from build123d import *

# Parameters (mm, degrees)
SKETCH_1_W                   = 20
SKETCH_1_H                   = 40
EXTRUDE_1_DEPTH              = 5.5
SKETCH_2_W                   = 2
SKETCH_2_H                   = 2
CUT_EXTRUDE_1_DEPTH          = 46.058295574
SKETCH_3_R                   = 2.25
EXTRUDE_2_DEPTH              = 40
SKETCH_3_2_R                 = 2.25
CUT_EXTRUDE_2_DEPTH          = 46.82575695
CHAMFER_1_SIZE               = 2
SKETCH_4_W                   = 9
SKETCH_4_H                   = 10
CUT_EXTRUDE_3_DEPTH          = 31
HOLE_WIZARD_M5_3_D           = 5.3
HOLE_WIZARD_M5_3_DEPTH       = 6
HOLE_WIZARD_M5_3_CSINK_D     = 10.2
HOLE_WIZARD_M5_3_CSINK_ANGLE = 70
HOLE_WIZARD_M5_3_TIP         = 1.59228064


with BuildPart() as part:
    # 草图1 → 凸台-拉伸1 (new body)
    with BuildSketch(Plane(origin=(0, 0, 0), x_dir=(1, 0, 0), z_dir=(0, 1, 0))):
        with Locations((-10, 0)):
            Rectangle(SKETCH_1_W, SKETCH_1_H)
    extrude(amount=EXTRUDE_1_DEPTH)

    # 草图2 → 切除-拉伸1 (cut, through all)
    with BuildSketch(Plane.XY.offset(20)):
        with Locations((-1, 1)):
            Rectangle(SKETCH_2_W, SKETCH_2_H)
    extrude(amount=-CUT_EXTRUDE_1_DEPTH, mode=Mode.SUBTRACT)

    # 草图3 → 凸台-拉伸2 (add)
    with BuildSketch(Plane.XY.offset(20)):
        with BuildLine():
            Line((-1.968626967, 10), (1.968626967, 10))
            Line((1.968626967, 10), (3.968626967, 8))
            Line((3.968626967, 8), (3.968626967, 5.5))
            ThreePointArc((3.968626967, 5.5), (0, 2), (-3.968626967, 5.5))
            Line((-3.968626967, 5.5), (-3.968626967, 8))
            Line((-3.968626967, 8), (-1.968626967, 10))
        make_face()
        with Locations((0, 6)):
            Circle(SKETCH_3_R, mode=Mode.SUBTRACT)
    extrude(amount=-EXTRUDE_2_DEPTH)

    # 草图3<2> → 切除-拉伸2 (cut, through all)
    with BuildSketch(Plane.XY.offset(20)):
        with Locations((0, 6)):
            Circle(SKETCH_3_2_R)
    extrude(amount=-CUT_EXTRUDE_2_DEPTH, mode=Mode.SUBTRACT)

    # 倒角1
    chamfer_1_edges = [part.edges().sort_by_distance(p)[0] for p in [
        (-20, 5.5, 0),
    ]]
    chamfer(chamfer_1_edges, length=CHAMFER_1_SIZE)

    # 草图4 → 切除-拉伸3 (cut, through all)
    with BuildSketch(Plane(origin=(0, 0, 0), x_dir=(1, 0, 0), z_dir=(0, 1, 0))):
        with Locations((-0.531373033, 5)):
            Rectangle(SKETCH_4_W, SKETCH_4_H)
        with Locations((-0.531373033, -15)):
            Rectangle(SKETCH_4_W, SKETCH_4_H)
    extrude(amount=CUT_EXTRUDE_3_DEPTH, mode=Mode.SUBTRACT)

    # M5 十字切槽平头螺钉锥孔槽口3
    with Locations(Plane(origin=(0, 5.5, 0), x_dir=(1, 0, 0), z_dir=(0, 1, 0))):
        with Locations((-12.5, 12.5), (-12.5, -12.5)):
            CounterSinkHole(HOLE_WIZARD_M5_3_D / 2, HOLE_WIZARD_M5_3_CSINK_D / 2, depth=HOLE_WIZARD_M5_3_DEPTH, counter_sink_angle=HOLE_WIZARD_M5_3_CSINK_ANGLE)
            with Locations((0, 0, -(HOLE_WIZARD_M5_3_DEPTH + HOLE_WIZARD_M5_3_TIP / 2))):  # 118° drill point
                Cone(0, HOLE_WIZARD_M5_3_D / 2, HOLE_WIZARD_M5_3_TIP, mode=Mode.SUBTRACT)


solid = part.part
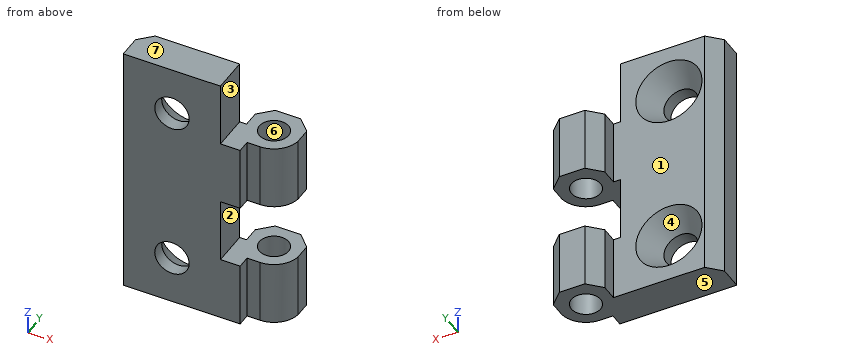
Read the model definition and answer for the solid it produces. Units are mm, in the model's axes. Face numbers are marked on the shaded views. A direction names the side the tool comes from. Give positions to 0.01 mm unless a question says otherwise; leave off trailing zeros. Write each loop counter-clockwise with the first axis right and the second up, starting at its lowest first coordinate (ties: lowest second). Pieces come first, ordered by that corner, then holes. Notation, with made-up numbers: (-12, 33.5) - (42, 33.5) arc R8 ccw to (42, 43.5) - close; hole circle Ø6 at (77.5, 70). An arc over 180 degrees is marked (long way). Use CSV: the item, a comma, the result in double quotes. Start each with the question number.
(1) Consider line 1 along Z through (x, y) = (-12.5, 1.6); line 2 along X through (y, z) = (6, -15.5); line 3 along Y through (x, z) = (0, 3.75). Determine where each line is inside the solid, lowest interval first.
(2) Find section C-C (x = -12.5). Give the vertices of the cut face in (y, z), plus the area to 3 significant figures.
(3) Given P1, Ø11, axis at x = -11.5, z = 5.5, coming from the +Y side; P2, Ø1.6, axis at y = 1.5, z = 6.5, coming from the +X side; P3, Ø1.6, axis at y = 1, z = -17.5, coming from the +X side, each flat-ended and moving along its own axis, determine where each tip first touches the part or whether it passes through.
(4) Find section B-B (y = 6). Give the vertices of the cut face in (x, z).
(5) Determine the mould class of the marked faces 4, 5, 6 and 7 for opening direction Z: +Z half, -Z half, draft (parallel to the pull), parting line (faces both ways), or undercut.
(6) For the marked faces 1, 2 and 3, determine the directions among +Z, -Z, +X, -X, +Y, -Y from which every point of the face is accessible in a straight line to the end or side of a thin tool.
(7) Find section A-A (z = 12.5). Give the vertices of the cut face in (x, y).
(8) Find section D-D (y = 8.75). Give the vertices of the cut face in (x, z), plus the area to 3 significant figures.
Findings below:
1,line 1,"-20 to -15.15, -9.85 to 9.85, 15.15 to 20"
1,line 2,"-3.97 to -2.25, 2.25 to 3.97"
1,line 3,"2 to 3.75, 8.25 to 10"
2,outline,"(0, -20) - (5.5, -20) - (5.5, -17.6) - (2, -15.15) - (0, -15.15) - close; (0, -9.85) - (2, -9.85) - (5.5, -7.4) - (5.5, 7.4) - (2, 9.85) - (0, 9.85) - close; (0, 15.15) - (2, 15.15) - (5.5, 17.6) - (5.5, 20) - (0, 20) - close"
2,area,"145 mm2"
3,P1,"y = 5.5"
3,P2,"x = 1.52"
3,P3,"x = -2"
4,outline,"(-3.97, -20) - (-2.25, -20) - (-2.25, -10) - (-3.97, -10) - close; (-3.97, 0) - (-2.25, 0) - (-2.25, 10) - (-3.97, 10) - close; (2.25, -20) - (3.97, -20) - (3.97, -10) - (2.25, -10) - close; (2.25, 0) - (3.97, 0) - (3.97, 10) - (2.25, 10) - close"
5,face 4,"undercut"
5,face 5,"-Z half"
5,face 6,"draft"
5,face 7,"+Z half"
6,face 1,"+Z, -Z, -X, +Y"
6,face 2,"+X, +Y, -Y"
6,face 3,"+Z, +X, +Y, -Y"
7,outline,"(-20, 0) - (-15.15, 0) - (-15.15, 2) - (-17.6, 5.5) - (-18, 5.5) - (-20, 3.5) - close; (-9.85, 0) - (-5.03, 0) - (-5.03, 5.5) - (-7.4, 5.5) - (-9.85, 2) - close"
8,outline,"(-3.22, -20) - (3.22, -20) - (3.22, -10) - (-3.22, -10) - close; (-3.22, 0) - (3.22, 0) - (3.22, 10) - (-3.22, 10) - close"
8,area,"129 mm2"
